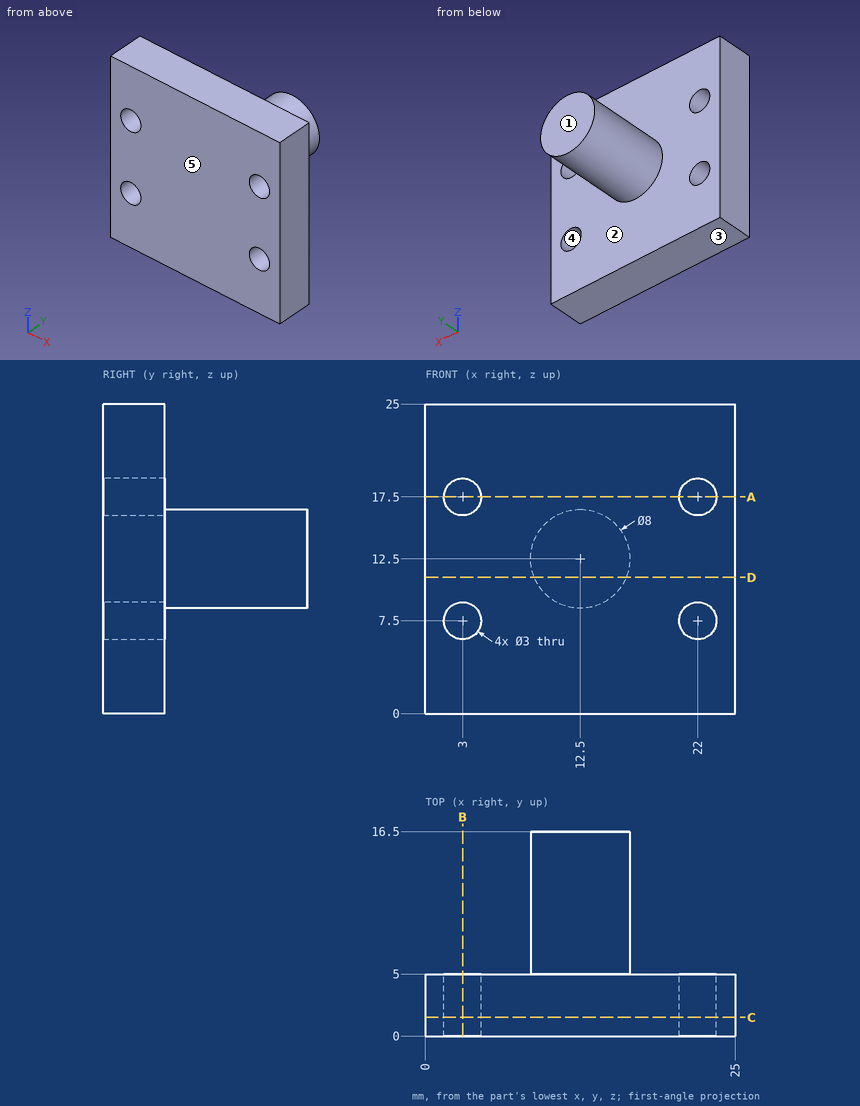
Part print with two shaded views. Sizes in mm from the minimum x, y, z corner. A direction names the side the tool comes from. Round coordinates to 2 decimals unless told otherwise and drop trailing zeros. Order: outer loops, then holes, each group sorted by start corner. A loop starts at its lowest first (then second) coordinate and runs counter-clockwise, first axis right, second up. Notation, with made-up numbers: M 15.5,-28 L 64.5,-28 A19 ccw 64.5,-1 Z; hole C -33.75,-8.75 d9. An arc over 180 degrees is marked long. Use CSV: the item, a comma, the result in double quotes. Start each with the question number.
(1) Cut at D-D on z = 11. List the corners of the cut face in (x, y), then the cut area to 3 significant figures.
(2) Cut at A-A on z = 17.5. List the corners of the cut face in (x, y), then the cut area to 3 significant figures.
(3) Drill centre lines: probe 1 along X at (y, z) = (1.9, 17.5); probe 2 along Z at (x, y) = (2.25, 4.5); probe 3 along Y at (x, z) = (20.5, 13). Where is each one in solid material? Low to high.
(4) Flat gauge pins, fed straight in: P1, Ø4, axis at x = 13, y = 4.5, coming from the -Z side; P2, Ø3.5, axis at x = 22, z = 17.5, coming from the +Y side; P3, Ø8, axis at x = 16, y = 9.5, coming from the -Z side; P4, Ø6, axis at x = 17.5, y = 9.5, coming from the -Z side. Where does each tip first touch, or does it go through?
(5) Mould opens along Z. For the marked faces 3, 4 and 5 say: +Z half, -Z half, draft (parallel to the pull), parting line (faces both ways), or undercut.
(6) Cut at C-C on y = 1.5. List the corners of the cut face in (x, z), then the cut area to 3 significant figures.
(7) Cut at B-B on x = 3. List the corners of the cut face in (y, z), then the cut area to 3 significant figures.
(8) Tool access for the marked faces 1 and 2: list every direction of +Z, -Z, +X, -X, +Y, -Y with a clear straight run to the whole face (end or side of a thin tool).
Findings:
1,outline,"M 0,0 L 25,0 L 25,5 L 16.21,5 L 16.21,16.5 L 8.79,16.5 L 8.79,5 L 0,5 Z"
1,area,"210 mm^2"
2,outline,"M 0,0 L 1.5,0 L 1.5,5 L 0,5 Z; M 4.5,0 L 20.5,0 L 20.5,5 L 4.5,5 Z; M 23.5,0 L 25,0 L 25,5 L 23.5,5 Z"
2,area,"95.0 mm^2"
3,probe 1,"x = 0 to 1.5, 4.5 to 20.5, 23.5 to 25"
3,probe 2,"z = 0 to 6.2, 8.8 to 16.2, 18.8 to 25"
3,probe 3,"y = 0 to 5"
4,P1,"stops at z = 0"
4,P2,"stops at y = 5"
4,P3,"stops at z = 8.5"
4,P4,"stops at z = 9.04"
5,face 3,"-Z half"
5,face 4,"undercut"
5,face 5,"draft"
6,outline,"M 0,0 L 25,0 L 25,25 L 0,25 Z; hole C 3,7.5 d3; hole C 3,17.5 d3; hole C 22,7.5 d3; hole C 22,17.5 d3"
6,area,"597 mm^2"
7,outline,"M 0,0 L 5,0 L 5,6 L 0,6 Z; M 0,9 L 5,9 L 5,16 L 0,16 Z; M 0,19 L 5,19 L 5,25 L 0,25 Z"
7,area,"95.0 mm^2"
8,face 1,"+Z, -Z, +X, -X, +Y"
8,face 2,"+Y"
